The model under review builds one solid part; all positions refer to its coordinate system, in mm. Give positions to 0.01 mm unless a question says otherwise; leave off trailing zeros. Loops run counter-clockwise (first coordinate to the right, second up) from the corner with the lowest first, then second, coordinate; pieces in that order, holes last. Notation, with made-up numbers: M 56.25,-33.5 L 95.25,-33.5 A21 cw 95.25,-28.5 Z; hole C -40,58 d8. An arc over 180 degrees is marked long. One line per item, written item: value. Start each with the question number.
Q1. We need section B-B on x = -40.5. Write out the cut boundary in (y, z) (3 decimals), plus the area to 3 significant figures.
Q2. To check wall thickness, follow line 1 along X through (y, z) = (14, 1.45); line 2 along Y through (x, z) = (-22, 0.75) (3 decimals); line 3 along X through (y, z) = (-47, 3). State the ranges of each line that lie inside material, in increasing order. Write a range as from..to.
Q3. We need section D-D on x = 42. Write out the cut boundary in (y, z) (3 decimals), plus the area to 3 significant figures.
Q4. We need section C-C on y = -26. Write out the cut boundary in (x, z) (3 decimals), plus the area to 3 significant figures.
Q5. We need section A-A on y = 57. Write out the cut boundary in (x, z) (3 decimals), plus the area to 3 significant figures.
Q6. For pin 1 (1 mm diameter, centred on x = 74, z = 2, fed in from +Y); pin 2 (1.6 mm diameter, centred on y = 65.5, z = 2, fed in from +X); pin 3 (1.6 mm diameter, centred on x = -0.5, z = 2, fed in from +Y); pin 4 (4 mm diameter, centred on x = 31, y = 37.5, fed in from -Z), all flat-tipped, find the tip position at first contact; note any pin that passes through.
```python
from build123d import *

# Parameters (mm, degrees)
F0_W     = 2.155658
F0_H     = 63.5
F0_W_2   = 76.2
F0_H_2   = 56.771246
F0_W_3   = 59.0296
F0_H_3   = 57.15
F0_W_4   = 3.81
F0_H_4   = 6.35
F0_W_5   = 25.4
F0_H_5   = 12.7
F1_DEPTH = 3.175


with BuildPart() as f1:
    # F0 (on Top) → F1 (new body)
    with BuildSketch(Plane.XY):
        with Locations((-1.077829, 31.75)):
            Rectangle(F0_W, F0_H)
        Polygon((0, 0), (-2.155658, 0), (-2.155658, 63.5), (-31.75, 63.5), (-72.005658, 63.5), (-72.005658, 0), (-31.75, 0), (-31.75, -66.675), (57.15, -66.675), (57.15, 0), (97.405658, 0), (97.405658, 63.5), (57.15, 63.5), (27.555658, 63.5), (27.555658, 0), (25.4, 0), (12.7, 0), align=None)
        with Locations((12.7, -31.939377)):
            Rectangle(F0_W_2, F0_H_2, mode=Mode.SUBTRACT)
        with Locations((-36.432958, 31.4579)):
            Rectangle(F0_W_3, F0_H_3, mode=Mode.SUBTRACT)
        with Locations((61.832958, 31.4579)):
            Rectangle(F0_W_3, F0_H_3, mode=Mode.SUBTRACT)
        Polygon((-31.75, 63.5), (-2.155658, 63.5), (0, 63.5), (0, 69.85), (-6.35, 69.85), (-31.75, 69.85), align=None)
        with Locations((1.905, 66.675)):
            Rectangle(F0_W_4, F0_H_4)
        with Locations((26.477829, 31.75)):
            Rectangle(F0_W, F0_H)
        with Locations((-19.05, 76.2)):
            Rectangle(F0_W_5, F0_H_5)
        Polygon((25.4, 69.85), (25.4, 63.5), (27.555658, 63.5), (57.15, 63.5), (57.15, 69.85), (31.75, 69.85), align=None)
        with Locations((23.495, 66.675)):
            Rectangle(F0_W_4, F0_H_4)
        with Locations((44.45, 76.2)):
            Rectangle(F0_W_5, F0_H_5)
    extrude(amount=F1_DEPTH)


solid = f1.part
```
Solved:
1. outline: M 0,0 L 2.883,0 L 2.883,3.175 L 0,3.175 Z; M 60.033,0 L 63.5,0 L 63.5,3.175 L 60.033,3.175 Z
1. area: 20.2 mm2
2. line 1: -72.01..-65.95, -6.92..0, 25.4..32.32, 91.35..97.41
2. line 2: -66.675..-60.325, -3.554..2.883, 60.033..82.55
2. line 3: -31.75..-25.4, 50.8..57.15
3. outline: M -66.675,0 L -60.325,0 L -60.325,3.175 L -66.675,3.175 Z; M -3.554,0 L 2.883,0 L 2.883,3.175 L -3.554,3.175 Z; M 60.033,0 L 82.55,0 L 82.55,3.175 L 60.033,3.175 Z
3. area: 112 mm2
4. outline: M -31.75,0 L -25.4,0 L -25.4,3.175 L -31.75,3.175 Z; M 50.8,0 L 57.15,0 L 57.15,3.175 L 50.8,3.175 Z
4. area: 40.3 mm2
5. outline: M -72.006,0 L -65.948,0 L -65.948,3.175 L -72.006,3.175 Z; M -6.918,0 L 0,0 L 0,3.175 L -6.918,3.175 Z; M 25.4,0 L 32.318,0 L 32.318,3.175 L 25.4,3.175 Z; M 91.348,0 L 97.406,0 L 97.406,3.175 L 91.348,3.175 Z
5. area: 82.4 mm2
6. pin 1: y = 63.5
6. pin 2: x = 57.15
6. pin 3: y = 69.85
6. pin 4: z = 0
